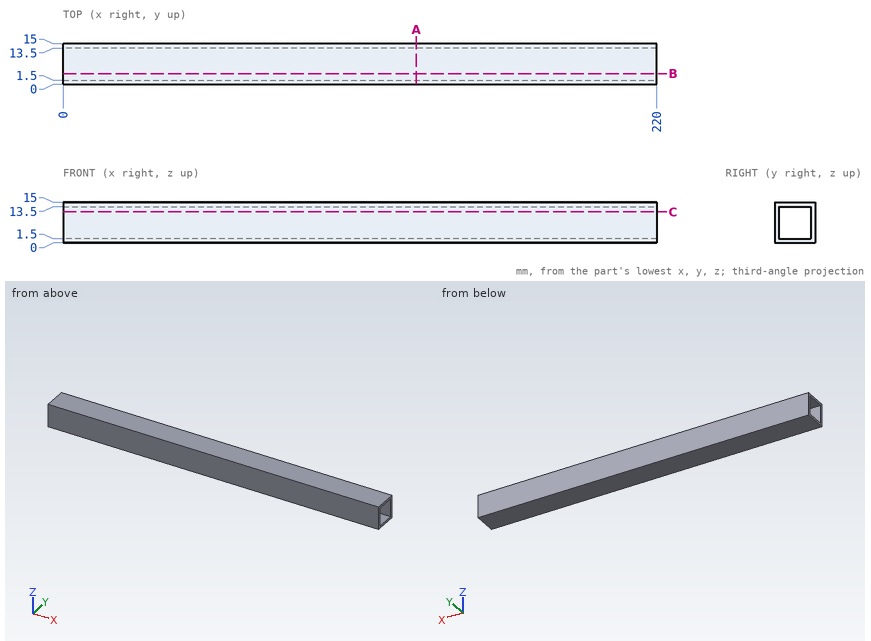
Input: dimensioned drawing with shaded views. Units: mm. Origin: part minimum x, y, z. Give positions to 0.01 mm unless a question says otherwise; leave off trailing zeros. Order: outer loops, then holes, each group sorted by start corner. A loop starts at its lowest first (then second) coordinate and runs counter-clockwise, first axis right, second up.
(1) Section query A-A (x = 131). Return the cut outline in (y, z), plus the area to 3 significant figures.
(2) Material intervals for line 1 along Z through (x, y) = (128.5, 12.5), sorted ascending.
(3) Section query B-B (y = 4). Return the cut outline in (x, z).
Outcome:
1. outline: (0, 0) - (15, 0) - (15, 15) - (0, 15) - close; hole (1.5, 1.5) - (13.5, 1.5) - (13.5, 13.5) - (1.5, 13.5) - close
1. area: 81.0 mm2
2. line 1: z = 0 to 1.5, 13.5 to 15
3. outline: (0, 0) - (220, 0) - (220, 1.5) - (0, 1.5) - close; (0, 13.5) - (220, 13.5) - (220, 15) - (0, 15) - close
